from build123d import *

# Parameters (mm, degrees)
SKETCH_1_W          = 47
SKETCH_1_H          = 35.6
EXTRUDE_1_DEPTH     = 59
SKETCH_3_W          = 59
SKETCH_3_H          = 32.6
CUT_EXTRUDE_1_DEPTH = 43
SKETCH_4_R          = 2.5
SKETCH_4_W          = 20
SKETCH_4_H          = 40
CUT_EXTRUDE_2_DEPTH = 49
SKETCH_6_R          = 2
CUT_EXTRUDE_3_DEPTH = 10


with BuildPart() as part:
    # 草图1 → 凸台-拉伸1 (new body)
    with BuildSketch(Plane.XY):
        with Locations((23.5, 17.8)):
            Rectangle(SKETCH_1_W, SKETCH_1_H)
    extrude(amount=EXTRUDE_1_DEPTH)

    # 草图3 → 切除-拉伸1 (cut)
    with BuildSketch(Plane.ZY):
        with Locations((29.5, 16.3)):
            Rectangle(SKETCH_3_W, SKETCH_3_H)
    extrude(amount=-CUT_EXTRUDE_1_DEPTH, mode=Mode.SUBTRACT)

    # 草图4 → 切除-拉伸2 (cut)
    with BuildSketch(Plane.XZ.offset(-32.6)):
        with Locations(Location((3.9, 54.25, 0), (0, 0, 270))):
            Circle(SKETCH_4_R)
        with Locations(Location((13.9, 54.25, 0), (0, 0, 270))):
            Circle(SKETCH_4_R)
        with Locations(Location((13.9, 4.75, 0), (0, 0, 270))):
            Circle(SKETCH_4_R)
        with Locations(Location((3.9, 4.75, 0), (0, 0, 270))):
            Circle(SKETCH_4_R)
        with Locations((10, 29.5)):
            Rectangle(SKETCH_4_W, SKETCH_4_H)
    extrude(amount=-CUT_EXTRUDE_2_DEPTH, mode=Mode.SUBTRACT)

    # 草图6 → 切除-拉伸3 (cut)
    with BuildSketch(Plane.ZY.offset(-43)):
        with Locations((43.5, 26.6)):
            Circle(SKETCH_6_R)
        with Locations((15.5, 26.6)):
            Circle(SKETCH_6_R)
        with Locations((43.5, 10.1)):
            Circle(SKETCH_6_R)
        with Locations((15.5, 10.1)):
            Circle(SKETCH_6_R)
    extrude(amount=-CUT_EXTRUDE_3_DEPTH, mode=Mode.SUBTRACT)


solid = part.part
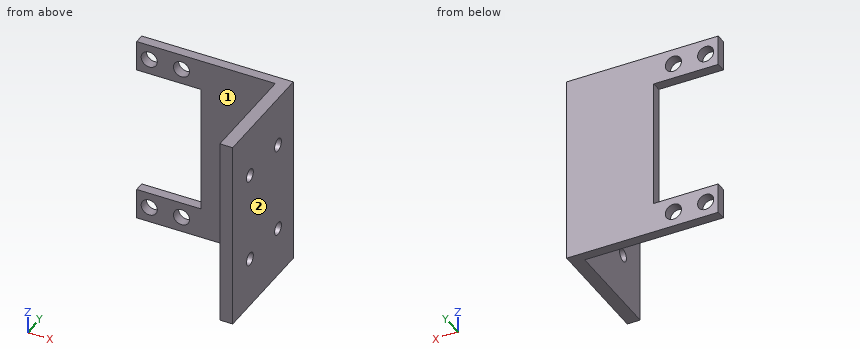
Can you work these out from the model? Positions are in its coordinate system, mm. Face numbers are marked on the shaded views. A direction names the side the tool comes from. Give positions to 0.01 mm unless a question says otherwise; leave off trailing zeros. Loops run counter-clockwise (first coordinate to the right, second up) from the corner with the lowest first, then second, coordinate; pieces in that order, holes last. Notation, with made-up numbers: (20, -14.5) -> (72, -14.5) arc R9 ccw to (72, 2.5) -> close; hole circle Ø3 at (-24, 0). An arc over 180 degrees is marked (long way). Return JSON: item names as keys, results as strings.
Q1. On a 3-axis mill with a long thin cutter (end or side, diameter ignored), from which of +Z, -Z, +X, -X, +Y, -Y can I reach the whole of each face in a straight line? I mean the marked faces 1 and 2. Say none if no direction works.
Checks:
{"face 1": "+Z, -Z, -X, -Y", "face 2": "+Z, -Z, +X, +Y, -Y"}
Q2. I want a section at A-A, the plane x = 8. List the corners of the cut face in (y, z) for me.
Checks:
{"outline": "(32.6, 0) -> (35.6, 0) -> (35.6, 9.5) -> (32.6, 9.5) -> close; (32.6, 49.5) -> (35.6, 49.5) -> (35.6, 59) -> (32.6, 59) -> close"}
Q3. I want a section at C-C, the plane y = 26.6. List the corners of the cut face in (x, z) for me, then the cut area to 3 significant figures.
Checks:
{"outline": "(43, 0) -> (47, 0) -> (47, 13.5) -> (43, 13.5) -> close; (43, 17.5) -> (47, 17.5) -> (47, 41.5) -> (43, 41.5) -> close; (43, 45.5) -> (47, 45.5) -> (47, 59) -> (43, 59) -> close", "area": "204 mm2"}
Q4. I need wall thicknesses on probe 1 along X at (y, z) = (33.25, 54.25); probe 2 along Y at (x, z) = (44, 43); probe 3 along Y at (x, z) = (46, 15.5). Which ranges of each line are inside material? Lowest first, please.
Checks:
{"probe 1": "x = 0 to 1.4, 6.4 to 11.4, 16.4 to 47", "probe 2": "y = 0 to 8.16, 12.04 to 24.66, 28.54 to 35.6", "probe 3": "y = 0 to 8.1, 12.1 to 24.6, 28.6 to 35.6"}
Q5. I want a section at B-B, the plane z = 54.25. List the corners of the cut face in (x, y) for me, then the cut area to 3 significant figures.
Checks:
{"outline": "(0, 32.6) -> (1.4, 32.6) -> (1.4, 35.6) -> (0, 35.6) -> close; (6.4, 32.6) -> (11.4, 32.6) -> (11.4, 35.6) -> (6.4, 35.6) -> close; (16.4, 32.6) -> (43, 32.6) -> (43, 0) -> (47, 0) -> (47, 35.6) -> (16.4, 35.6) -> close", "area": "241 mm2"}
Q6. For pin 1 Ø3 at (x, z) = (13.9, 54.25) entering from +Y; pin 2 Ø2.5 at (y, z) = (34.5, 24) entering from -X; pin 3 Ø16.5 at (y, z) = (16.5, 21.5) entering from -X; pin 4 Ø6.5 at (x, z) = (13.9, 4.75) entering from -Y, each with a flat end and sliding along its axis, tell me the tip position at first contact or that it passes through.
Checks:
{"pin 1": "passes through", "pin 2": "stops at x = 20", "pin 3": "stops at x = 43", "pin 4": "stops at y = 32.6"}
Q7. I want a section at D-D, the plane z = 38.5. List the corners of the cut face in (x, y) for me.
Checks:
{"outline": "(20, 32.6) -> (43, 32.6) -> (43, 0) -> (47, 0) -> (47, 35.6) -> (20, 35.6) -> close"}
